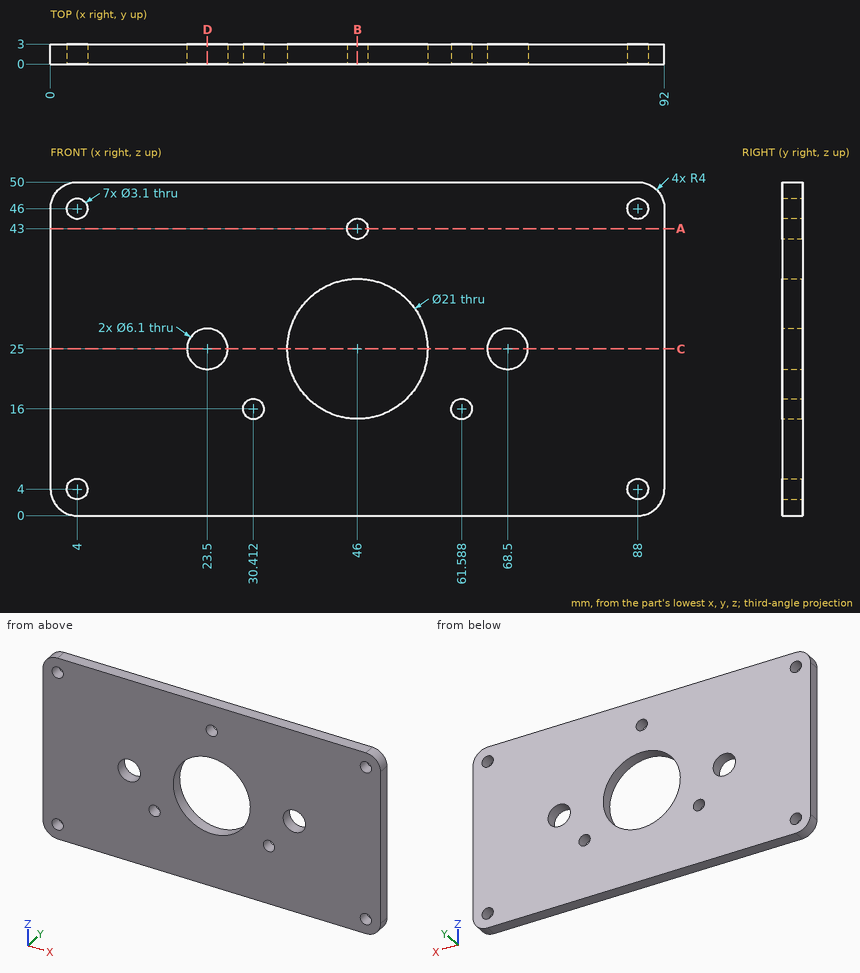
Could you check a few things on this drawing? It's one solid part, dimensions in mm from its lowest x, y, z. Coordinates: 2 decimals unless noted, no trailing zeros. Order: outer loops, then holes, each group sorted by start corner. A loop starts at its lowest first (then second) coordinate and runs counter-clockwise, first axis right, second up. Notation, with made-up numbers: M 83,-25 L 117,-25 A14 cw 117,-6 Z; hole C -0.75,51 d8. An arc over 180 degrees is marked long. Use a Markdown table: item, result. Add a question column.
Q1. I want a section at A-A on z = 43. List the corners of the cut face in (x, y) for me, then the cut area to 3 significant figures.
Q2. I'm going to push a flat-ended pin straight in: pin 1 (1.5 mm diameter, centred on x = 21.5, y = 1, fed in from -Z). Where does the tip first touch, or does it pass through?
Q3. If I drill on L1, parallel to X at y = 1.5, z = 4; L2, parallel to X at y = 0.2, z = 3 (1 decimal); L3, parallel to X at y = 1.45, z = 16 (1 decimal), over which ranges is the centre line in solid material (lowest first)?
Q4. I want a section at B-B on x = 46. List the corners of the cut face in (y, z) for me.
Q5. I want a section at D-D on x = 23.5. List the corners of the cut face in (y, z) for me.
Q6. I want a section at C-C on z = 25. List the corners of the cut face in (x, y) for me.
Checked values:
| question | item | result |
|---|---|---|
| 1 | outline | M 0,0 L 44.45,0 L 44.45,3 L 0,3 Z; M 47.55,0 L 92,0 L 92,3 L 47.55,3 Z |
| 1 | area | 267 mm² |
| 2 | pin 1 | z = 0 |
| 3 | L1 | 0 to 2.45, 5.55 to 86.45, 89.55 to 92 |
| 3 | L2 | 0.1 to 2.8, 5.2 to 86.8, 89.2 to 91.9 |
| 3 | L3 | 0 to 28.9, 32 to 40.6, 51.4 to 60, 63.1 to 92 |
| 4 | outline | M 0,0 L 3,0 L 3,14.5 L 0,14.5 Z; M 0,35.5 L 3,35.5 L 3,41.45 L 0,41.45 Z; M 0,44.55 L 3,44.55 L 3,50 L 0,50 Z |
| 5 | outline | M 0,0 L 3,0 L 3,21.95 L 0,21.95 Z; M 0,28.05 L 3,28.05 L 3,50 L 0,50 Z |
| 6 | outline | M 0,0 L 20.45,0 L 20.45,3 L 0,3 Z; M 26.55,0 L 35.5,0 L 35.5,3 L 26.55,3 Z; M 56.5,0 L 65.45,0 L 65.45,3 L 56.5,3 Z; M 71.55,0 L 92,0 L 92,3 L 71.55,3 Z |
